The listing builds one solid part. Answer for the finished solid, in the listing's coordinates (mm). A direction names the side the tool comes from. Give positions to 0.01 mm unless a question says otherwise; leave off trailing zeros. Order: outer loops, then holes, each group sorted by start corner. A loop starts at its lowest first (then second) coordinate and runs counter-clockwise, first axis right, second up. Notation, with made-up numbers: (55.25, -28) - (95.25, -28) arc R22 ccw to (95.25, -21) - close; hole circle Ø11 at (83, 17.25). An arc over 180 degrees is marked (long way). Use a Markdown table: item, result. Add a question column.
1) Find section C-C, the plane y = -24.5. Determine the outline of the cut face in (x, z).
2) Straight lines are drawn through the part: line 1 (X direction, y = -48, z = 11); line 2 (Z direction, x = -11.5, y = -14); line 3 (Z direction, x = -6, y = -13). For each, find the intervals that lie inside material, in ascending order.
3) For faces 5 (the face through (-10, -25, -4)), 6 (the face through (-13, -25, -25)), determine the directions among +Z, -Z, +X, -X, +Y, -Y from which every point of the face is accessible in a straight line to the end or side of a thin tool.
4) The mould has two halves that part along Y. Classify faces 1 (the face through (-10.2, 0, 5.9)), 2 (the face through (-10.2, -50, 5.9)), 3 (the face through (-14, -25, 23)), 4 (the face through (-12.465, -6.777, 1.802)): released by +Y, released by -Y, zero draft, split by the parting line, or undercut.
5) Find section D-D, the plane z = 0. Determine the outline of the cut face in (x, y).
6) Find section A-A, the plane z = -14. Determine the outline of the cut face in (x, y), plus the area to 3 significant figures.
7) Find section B-B, the plane y = -37.5. Determine the outline of the cut face in (x, z), plus the area to 3 significant figures.
8) Flat-ended cylindrical pins translate along their axes: pin 1 (21.5 mm diameter, centred on y = -37, z = 0.5, fed in from -X); pin 2 (4 mm diameter, centred on x = 0, y = -44, fed in from -Z). Find the tip coordinate at first contact, or state that the pin passes through.
from build123d import *

# Parameters (mm, degrees)
F1_DEPTH = 50
F2_R     = 6
F3_DEPTH = 30
F4_R     = 2
F5_R     = 5


with BuildPart() as f1:
    # F0 (on Front) → F1 (new body)
    with BuildSketch(Plane.XZ):
        Polygon((15, -25), (15, 25), (-15, 25), (-15, -25), (-10, -25), (-10, 20), (10, 20), (10, -25), align=None)
    extrude(amount=F1_DEPTH)

    # F2 (on face) → F3 (cut, through all)
    with BuildSketch(Plane.YZ.offset(15)):
        with Locations((-37.5, 0)):
            Circle(F2_R)
        with Locations((-12.5, 0)):
            Circle(F2_R)
    extrude(amount=-F3_DEPTH, mode=Mode.SUBTRACT)

    # F4
    f4_edges = [f1.edges().sort_by_distance(p)[0] for p in [
        (-10, -25, 20),
        (10, -25, 20),
    ]]
    fillet(f4_edges, radius=F4_R)

    # F5
    f5_edges = [f1.edges().sort_by_distance(p)[0] for p in [
        (15, -25, 25),
        (-15, -25, 25),
    ]]
    fillet(f5_edges, radius=F5_R)


solid = f1.part
The answers:
| question | item | result |
|---|---|---|
| 1 | outline | (-15, -25) - (-10, -25) - (-10, 18) arc R2 cw to (-8, 20) - (8, 20) arc R2 cw to (10, 18) - (10, -25) - (15, -25) - (15, 20) arc R5 ccw to (10, 25) - (-10, 25) arc R5 ccw to (-15, 20) - close |
| 2 | line 1 | -15 to -10, 10 to 15 |
| 2 | line 2 | -25 to -5.81, 5.81 to 24.77 |
| 2 | line 3 | 20 to 25 |
| 3 | face 5 | -Z, +Y, -Y |
| 3 | face 6 | -Z, +X, -X, +Y, -Y |
| 4 | face 1 | released by +Y |
| 4 | face 2 | released by -Y |
| 4 | face 3 | zero draft |
| 4 | face 4 | undercut |
| 5 | outline | (-15, -50) - (-10, -50) - (-10, -43.5) - (-15, -43.5) - close; (-15, -31.5) - (-10, -31.5) - (-10, -18.5) - (-15, -18.5) - close; (-15, -6.5) - (-10, -6.5) - (-10, 0) - (-15, 0) - close; (10, -50) - (15, -50) - (15, -43.5) - (10, -43.5) - close; (10, -31.5) - (15, -31.5) - (15, -18.5) - (10, -18.5) - close; (10, -6.5) - (15, -6.5) - (15, 0) - (10, 0) - close |
| 6 | outline | (-15, -50) - (-10, -50) - (-10, 0) - (-15, 0) - close; (10, -50) - (15, -50) - (15, 0) - (10, 0) - close |
| 6 | area | 500 mm2 |
| 7 | outline | (-15, -25) - (-10, -25) - (-10, -6) - (-15, -6) - close; (-15, 6) - (-10, 6) - (-10, 18) arc R2 cw to (-8, 20) - (8, 20) arc R2 cw to (10, 18) - (10, 6) - (15, 6) - (15, 20) arc R5 ccw to (10, 25) - (-10, 25) arc R5 ccw to (-15, 20) - close; (10, -25) - (15, -25) - (15, -6) - (10, -6) - close |
| 7 | area | 471 mm2 |
| 8 | pin 1 | x = -15 |
| 8 | pin 2 | z = 20 |
